Design review of the part built by this model. Coordinates are the model's own, in mm. Face numbers are marked on the shaded views. A direction names the side the tool comes from. Round coordinates to 2 decimals unless told otherwise and drop trailing zeros. Loops run counter-clockwise (first coordinate to the right, second up) from the corner with the lowest first, then second, coordinate; pieces in that order, holes last. Notation, with made-up numbers: (56, 17) - (110, 17) arc R30 cw to (110, 47) - close; hole circle Ø4 at (38.25, -16.75). An arc over 180 degrees is marked (long way). Return JSON: item names as keys, results as strings. Group by question number.
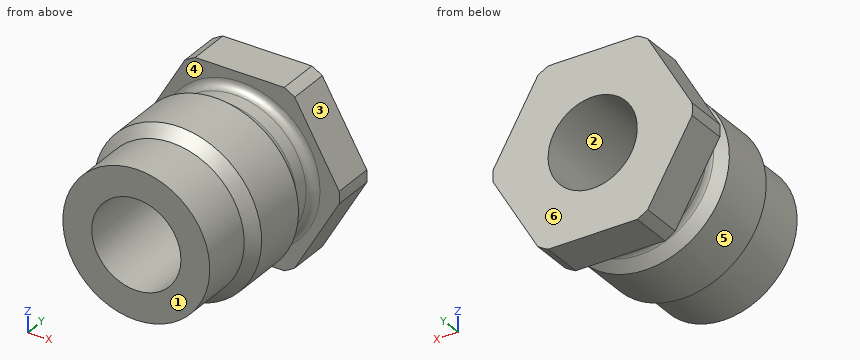
from build123d import *

# Parameters (mm, degrees)
SKETCH_2_OUTSIDE_W  = 27.582
SKETCH_2_OUTSIDE_H  = 27.582
CUT_EXTRUDE_1_DEPTH = 24.270152556


with BuildPart() as part:
    # Эскиз1 → Повернуть1 (revolve)
    with BuildSketch(Plane.XY, mode=Mode.PRIVATE) as revolve_1_sk:
        with BuildLine():
            Line((-4.25, 0), (-7, 0))
            Line((-7, 0), (-7, 5))
            Line((-7, 5), (-8, 6))
            Line((-8, 6), (-8, 11.35))
            Line((-8, 11.35), (-7.084314575, 12.265685425))
            ThreePointArc((-7.084314575, 12.265685425), (-6.910896374, 12.525224104), (-6.85, 12.83137085))
            Line((-6.85, 12.83137085), (-6.85, 14.2))
            ThreePointArc((-6.85, 14.2), (-7.084314575, 14.765685425), (-7.65, 15))
            Line((-7.65, 15), (-9.5, 15))
            Line((-9.5, 15), (-9.5, 19))
            Line((-9.5, 19), (-4.25, 19))
            Line((-4.25, 19), (-4.25, 0))
        make_face()
    revolve(revolve_1_sk.sketch.rotate(Axis((0, 0, 0), (0, 1, 0)), 270), axis=Axis((0, 0, 0), (0, 1, 0)))

    # Эскиз2 outside → Вырез-Вытянуть1 (cut, through all)
    with BuildSketch(Plane(origin=(0, 19, 0), x_dir=(1, 0, 0), z_dir=(0, 1, 0))):
        Rectangle(SKETCH_2_OUTSIDE_W, SKETCH_2_OUTSIDE_H)
        Polygon((9.814954576, 0), (4.907477288, 8.5), (-4.907477288, 8.5), (-9.814954576, 0), (-4.907477288, -8.5), (4.907477288, -8.5), align=None, mode=Mode.SUBTRACT)
    extrude(amount=-CUT_EXTRUDE_1_DEPTH, mode=Mode.SUBTRACT)


solid = part.part
Q1. Add section C-C, the plane y = 17.25. State the section outline as (x, z) points.
Q2. Add section D-D, the plane y = 13.25. State the section outline as (x, z) points, plus the area to 3 significant figures.
Q3. Insertion check: pin 1 Ø8 at (x, z) = (-2, 0) entering from -Y; pin 2 Ø10 at (x, y) = (-6, 10) entering from +Z; pin 3 Ø1 at (y, z) = (8, 0.5) entering from +X. Each pin has a flat end and moves straight along its axis. Give the tip position at first contact, or say it passes through.
Q4. Draft analysis for pull direction X (two halves, no side actions). For the marked faces 1, 2 and 3, state which applies: pulls with the +X half, pulls with the -X half, needs draft (parallel to the pull), parting line crosses it, or undercut.
Q5. For line 1 (Z direction, x = -1, y = 16); line 2 (Y direction, x = 2, z = 7.5); line 3 (Y direction, x = 7, z = 3.75), list the stretches that pass through material, from the lowest coordinate up.
Q6. Add section A-A, the plane x = 0. State the section outline as (y, z) points, plus the area to 3 significant figures.
Q7. Add section B-B, the plane z = 0. State the section outline as (x, y) points, plus the area to 3 significant figures.
Q8. Tool access review of the marked faces 4, 5 and 6: name each direction out of +Z, -Z, +X, -X, +Y, -Y from which nothing blocks a thin tool from reaching the whole face with its end or side.
Evaluation:
{
 "1": {"outline": "(-9.48, -0.58) - (-5.24, -7.92) arc R9.5 ccw to (-4.24, -8.5) - (4.24, -8.5) arc R9.5 ccw to (5.24, -7.92) - (9.48, -0.58) arc R9.5 ccw to (9.48, 0.58) - (5.24, 7.92) arc R9.5 ccw to (4.24, 8.5) - (-4.24, 8.5) arc R9.5 ccw to (-5.24, 7.92) - (-9.48, 0.58) arc R9.5 ccw to start; hole circle Ø8.5 at (0, 0)"},
 "2": {"outline": "circle Ø13.7 at (0, 0); hole circle Ø8.5 at (0, 0)", "area": "90.7 mm²"},
 "3": {"pin 1": "y = 0", "pin 2": "z = 7.94", "pin 3": "x = 8"},
 "4": {"face 1": "needs draft", "face 2": "undercut", "face 3": "pulls with the +X half"},
 "5": {"line 1": "-8.5 to -4.13, 4.13 to 8.5", "line 2": "5.76 to 11.59, 15 to 19", "line 3": "5.94 to 11.41, 15 to 19"},
 "6": {"outline": "(0, -7) - (5, -7) - (6, -8) - (11.35, -8) - (12.27, -7.08) arc R0.8 cw to (12.83, -6.85) - (14.2, -6.85) arc R0.8 cw to (15, -7.65) - (15, -8.5) - (19, -8.5) - (19, -4.25) - (0, -4.25) - close; (0, 4.25) - (19, 4.25) - (19, 8.5) - (15, 8.5) - (15, 7.65) arc R0.8 cw to (14.2, 6.85) - (12.83, 6.85) arc R0.8 cw to (12.27, 7.08) - (11.35, 8) - (6, 8) - (5, 7) - (0, 7) - close", "area": "129 mm²"},
 "7": {"outline": "(-9.5, 15) - (-7.65, 15) arc R0.8 cw to (-6.85, 14.2) - (-6.85, 12.83) arc R0.8 cw to (-7.08, 12.27) - (-8, 11.35) - (-8, 6) - (-7, 5) - (-7, 0) - (-4.25, 0) - (-4.25, 19) - (-9.5, 19) - close; (4.25, 0) - (7, 0) - (7, 5) - (8, 6) - (8, 11.35) - (7.08, 12.27) arc R0.8 cw to (6.85, 12.83) - (6.85, 14.2) arc R0.8 cw to (7.65, 15) - (9.5, 15) - (9.5, 19) - (4.25, 19) - close", "area": "137 mm²"},
 "8": {"face 4": "none", "face 5": "-Y", "face 6": "+Z, -Z, +X, -X, +Y"}
}
